Geometry: final body of the model. Coordinates: model frame, mm. Face numbers are marked on the shaded views. A direction names the side the tool comes from. Give positions to 0.01 mm unless a question says otherwise; leave off trailing zeros. Loops run counter-clockwise (first coordinate to the right, second up) from the corner with the lowest first, then second, coordinate; pieces in that order, holes last. Notation, with made-up numbers: (16, 10.25) - (37, 10.25) arc R26 ccw to (37, 36.25) - close; hole circle Ø1 at (63.25, 0.5). An arc over 180 degrees is marked (long way). Use one line per item in the form item = value.
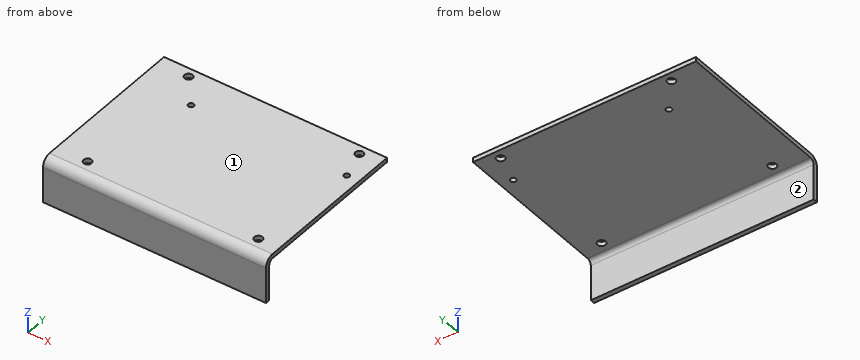
```python
from build123d import *

# Parameters (mm, degrees)
SKETCH1_W                    = 100
SKETCH1_H                    = 20
BASE_FLANGE1_DEPTH           = 2
EDGE_FLANGE1_STRIP_W         = 12
EDGE_FLANGE1_STRIP_H         = 2
EDGE_FLANGE1_STRIP_CUT_DEPTH = 100
EDGE_FLANGE1_DEPTH           = 100
M3_5_CLEARANCE_HOLE1_D       = 2.5
M3_CLEARANCE_HOLE1_D         = 3.6


# Sheet-metal steps are written as plain solids
with BuildPart() as part:
    # Sketch1 → Base-Flange1 (new body)
    with BuildSketch(Plane(origin=(0, 0, 0), x_dir=(1, 0, 0), z_dir=(0, 1, 0))):
        Rectangle(SKETCH1_W, SKETCH1_H)
    extrude(amount=-BASE_FLANGE1_DEPTH)

    # Edge-Flange1 strip (across the edge) → Edge-Flange1 strip cut (cut)
    with BuildSketch(Plane(origin=(-50, 0, 10), x_dir=(0, 0, -1), z_dir=(1, 0, 0))):
        with Locations((-2, -1)):
            Rectangle(EDGE_FLANGE1_STRIP_W, EDGE_FLANGE1_STRIP_H)
    extrude(amount=EDGE_FLANGE1_STRIP_CUT_DEPTH, mode=Mode.SUBTRACT)

    # Edge-Flange1 section (across the edge) → Edge-Flange1 (add)
    with BuildSketch(Plane(origin=(-50, 0, 10), x_dir=(0, 0, -1), z_dir=(1, 0, 0))):
        with BuildLine():
            Line((0, 2), (0, 72))
            Line((0, 72), (2, 72))
            Line((2, 72), (2, 2))
            ThreePointArc((2, 2), (2.585786438, 0.585786438), (4, 0))
            Line((4, 0), (4, -2))
            ThreePointArc((4, -2), (1.171572875, -0.828427125), (0, 2))
        make_face()
    extrude(amount=EDGE_FLANGE1_DEPTH)

    # M3.5 Clearance Hole1 (through all)
    with Locations(Plane(origin=(114.471522339, -206.957964235, 10), x_dir=(1, 0, 0), z_dir=(0, 0, 1))):
        with Locations((-139.871522339, 261.957964236), (-70.071522339, 261.957964236)):
            Hole(M3_5_CLEARANCE_HOLE1_D / 2)

    # M3 Clearance Hole1 (through all)
    with Locations(Plane(origin=(114.471522339, -206.957964235, 8), x_dir=(1, 0, 0), z_dir=(0, 0, -1))):
        with Locations((-150.471522339, -274.892964235), (-73.871522339, -274.892964235), (-73.871522339, -213.172964235), (-150.471522339, -213.172964235)):
            Hole(M3_CLEARANCE_HOLE1_D / 2)


solid = part.part
```
(1) Cut plane B-B (y = 55). Return the cut outline in (x, z).
Solution:
outline = (-50, 8) - (-26.65, 8) - (-26.65, 10) - (-50, 10) - close; (-24.15, 8) - (43.15, 8) - (43.15, 10) - (-24.15, 10) - close; (45.65, 8) - (50, 8) - (50, 10) - (45.65, 10) - close
(2) Cut plane C-C (x = -25.4). Return the cut outline in (y, z).
Solution:
outline = (-2, -10) - (0, -10) - (0, 6) arc R2 cw to (2, 8) - (53.75, 8) - (53.75, 10) - (2, 10) arc R4 ccw to (-2, 6) - close; (56.25, 8) - (72, 8) - (72, 10) - (56.25, 10) - close
(3) Access query for the marked faces 1 and 2. Directions: +Z, -Z, +X, -X, +Y, -Y. A direction counts if a zero-diameter tool reaches every point of the face in a straight line with its end or side. Return the directions, or none.
Solution:
face_1 = +Z, +X, -X, +Y, -Y
face_2 = -Z, +X, -X, +Y
(4) Material intervals for L1, parallel to Y at x = 40.6, z = 9.35 (3 decimals); L2, parallel to Z at x = 28, y = 62; L3, parallel to Y at x = 38.5, z = -3, sorted ascending. Write a range as from..to.
Solution:
L1 = -0.186..4.415, 8.015..66.135, 69.735..72
L2 = 8..10
L3 = -2..0
(5) Cut plane D-D (x = 14.5). Return the cut outline in (y, z).
Solution:
outline = (-2, -10) - (0, -10) - (0, 6) arc R2 cw to (2, 8) - (72, 8) - (72, 10) - (2, 10) arc R4 ccw to (-2, 6) - close
(6) Pin query (flat end, axial travel): P1, Ø12, axis at x = -23.5, y = 62, coming from the -Z side; P2, Ø8, axis at x = 10, z = -1.5, coming from the +Y side. Return the tip coordinate at first contact, or that it passes through.
Solution:
P1 = 8
P2 = 0
(7) Cut plane A-A (x = 40.6). Return the cut outline in (y, z) (3 decimals).
Solution:
outline = (-2, -10) - (0, -10) - (0, 6) arc R2 cw to (2, 8) - (4.415, 8) - (4.415, 10) - (2, 10) arc R4 ccw to (-2, 6) - close; (8.015, 8) - (66.135, 8) - (66.135, 10) - (8.015, 10) - close; (69.735, 8) - (72, 8) - (72, 10) - (69.735, 10) - close
